Design review of the part built by this model. Coordinates are the model's own, in mm. Face numbers are marked on the shaded views. A direction names the side the tool comes from. Coordinates: 2 decimals unless noted, no trailing zeros. Order: outer loops, then holes, each group sorted by start corner. A loop starts at its lowest first (then second) coordinate and runs counter-clockwise, first axis right, second up. Notation, with made-up numbers: (42, 59) - (59, 59) arc R16 cw to (59, 68) - close; hole circle Ø9 at (-10.5, 51.25). An arc over 180 degrees is marked (long way). Write each question's results on one line, items separated by ' | '. Start each with the question number.
```python
from build123d import *

# Parameters (mm, degrees)
SKETCH_1_R          = 2
EXTRUDE_1_DEPTH     = 5
CUT_EXTRUDE_1_DEPTH = 1.75
FILLET_1_R          = 0.2
SKETCH_2_R          = 2.2
EXTRUDE_2_DEPTH     = 0.0005


with BuildPart() as part:
    # 草图1 → 凸台-拉伸1 (new, symmetric)
    with BuildSketch(Plane(origin=(0, 0, 0), x_dir=(1, 0, 0), z_dir=(0, 1, 0))):
        with Locations(Location((0, 0, 0), (0, 0, 270))):
            Circle(SKETCH_1_R)
    extrude(amount=EXTRUDE_1_DEPTH, both=True)

    # 草图3 → 切除-拉伸1 (cut)
    with BuildSketch(Plane(origin=(0, 5, 0), x_dir=(1, 0, 0), z_dir=(0, 1, 0))):
        Polygon((1.154700538, 0), (0.577350269, 1), (-0.577350269, 1), (-1.154700538, 0), (-0.577350269, -1), (0.577350269, -1), align=None)
    extrude(amount=-CUT_EXTRUDE_1_DEPTH, mode=Mode.SUBTRACT)

    # 圆角1
    fillet_1_edges = [part.edges().sort_by_distance(p)[0] for p in [
        (0.866025404, 5, 0.5),
        (0.866025404, 5, -0.5),
        (0, 5, -1),
        (-0.866025404, 5, -0.5),
        (-0.866025404, 5, 0.5),
        (0, 5, 1),
        (0, -5, -2),
        (0, 5, -2),
    ]]
    fillet(fillet_1_edges, radius=FILLET_1_R)

    # 草图2 → 凸台-拉伸2 (add, symmetric)
    with BuildSketch(Plane(origin=(0, 0, 0), x_dir=(1, 0, 0), z_dir=(0, 1, 0))):
        with Locations(Location((0, 0, 0), (0, 0, 270))):
            Circle(SKETCH_2_R)
    extrude(amount=EXTRUDE_2_DEPTH, both=True)


solid = part.part
```
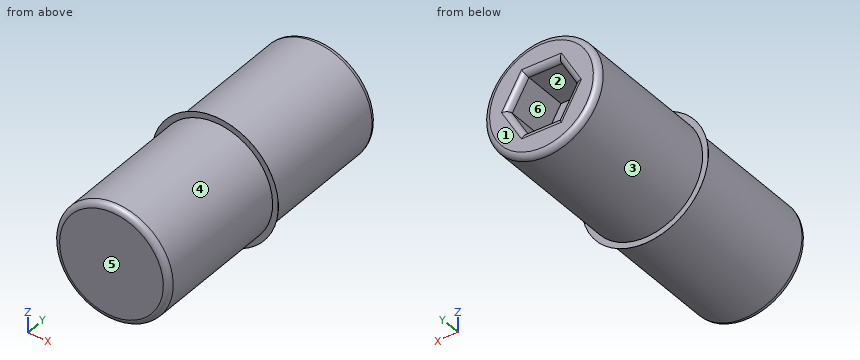
(1) Mouldability with a two-part tool opening along X and no side actions: class the marked faces 1, 2 and 3 as +X half, -X half, draft (parallel to the pull), parting line (faces both ways), or undercut.
(2) Take a section at A-A (y = 4.25). State the section outline as (x, z) points, plus the area to 3 significant figures.
(3) Take a section at C-C (y = 0.5). State the section outline as (x, z) points, plus the area to 3 significant figures.
(4) To check wall thickness, follow line 1 along Y through (x, z) = (0.4, 0.25); line 2 along X through (y, z) = (3.75, -0.3); line 3 along X through (y, z) = (0.5, -1.6). State the ranges of each line that lie inside material, in increasing order. Write a range as [from, to].
(5) Clearance check with a flat-ended pin moving along its axis: pin 1 (1.3 mm diameter, centred on x = 0, y = 3.5, fed in from +Z). State where the tip first meets the part, or that it passes through.
(6) Tool access review of the marked faces 4, 5 and 6: name each direction out of +Z, -Z, +X, -X, +Y, -Y from which nothing blocks a thin tool from reaching the whole face with its end or side.
Worked out:
1) face 1: draft | face 2: undercut | face 3: parting line
2) outline: circle Ø4 at (0, 0); hole (-1.15, 0) - (-0.58, -1) - (0.58, -1) - (1.15, 0) - (0.58, 1) - (-0.58, 1) - close | area: 9.10 mm^2
3) outline: circle Ø4 at (0, 0) | area: 12.6 mm^2
4) line 1: [-5, 3.25] | line 2: [-1.98, -0.98], [0.98, 1.98] | line 3: [-1.2, 1.2]
5) pin 1: z = 2
6) face 4: -Y | face 5: +Z, -Z, +X, -X, -Y | face 6: +Y
